Can you work these out from the model? Positions are in its coordinate system, mm. Give positions to 0.01 mm unless a question says otherwise; leave off trailing zeros. Order: outer loops, then holes, each group sorted by start corner. A loop starts at its lowest first (then second) coordinate and runs counter-clockwise, first axis right, second up. Notation, with made-up numbers: M 70,-33.75 L 108,-33.75 A29 cw 108,-1.75 Z; hole C 9.25,-19 d4. An arc over 180 degrees is marked long. Use one line per item in the form item = value. Start each with the question number.
1. I want a section at A-A, the plane z = 66.5. List the corners of the cut face in (x, y) for me.
2. I want a section at C-C, the plane x = 88.5. Count the separate pieces of the cut face and the enclosed holes in it, and give its area (3 significant figures).
3. Will these pins go through, and if not, where does the flat tip stop? P1, Ø2, axis at y = 2.5, z = 90.5, coming from the -X side; P2, Ø4, axis at x = -77.78, z = 77.78, coming from the +Y side; P3, Ø1, axis at y = 3.5, z = -82.5, coming from the -X side; P4, Ø1.5, axis at x = -49.5, y = 1, coming from the +Z side.
4. I want a section at B-B, the plane x = 8.5. List the corners of the cut face in (y, z) for me, and give its area (3 significant figures).
5. I need wall thicknesses on L1, parallel to Z at x = 86, y = 2; L2, parallel to Z at x = 0.5, y = 2; L3, parallel to X at y = 1.5, z = 76.5. Which ranges of each line are inside material? Lowest first, please.
```python
from build123d import *

# Parameters (mm, degrees)
SKETCH1_R           = 125
SKETCH1_R_2         = 1.5
BOSS_EXTRUDE1_DEPTH = 6


with BuildPart() as part:
    # Sketch1 → Boss-Extrude1 (new body)
    with BuildSketch(Plane(origin=(0, 0, 0), x_dir=(1, 0, 0), z_dir=(0, 1, 0))):
        with Locations(Location((0, 0, 0), (0, 0, 270))):
            Circle(SKETCH1_R)
        with Locations(Location((0, -110, 0), (0, 0, 270))):
            Circle(SKETCH1_R_2, mode=Mode.SUBTRACT)
        with Locations(Location((77.781745931, -77.781745931, 0), (0, 0, 270))):
            Circle(SKETCH1_R_2, mode=Mode.SUBTRACT)
        with Locations(Location((110, 0, 0), (0, 0, 270))):
            Circle(SKETCH1_R_2, mode=Mode.SUBTRACT)
        with Locations(Location((77.781745931, 77.781745931, 0), (0, 0, 270))):
            Circle(SKETCH1_R_2, mode=Mode.SUBTRACT)
        with Locations(Location((0, 110, 0), (0, 0, 90))):
            Circle(SKETCH1_R_2, mode=Mode.SUBTRACT)
        with Locations(Location((-77.781745931, 77.781745931, 0), (0, 0, 90))):
            Circle(SKETCH1_R_2, mode=Mode.SUBTRACT)
        with Locations(Location((-110, 0, 0), (0, 0, 90))):
            Circle(SKETCH1_R_2, mode=Mode.SUBTRACT)
        with Locations(Location((-77.781745931, -77.781745931, 0), (0, 0, 90))):
            Circle(SKETCH1_R_2, mode=Mode.SUBTRACT)
        with BuildLine():
            ThreePointArc((93.976500469, 13.907456977), (-95, 0), (93.976500469, -13.907456977))
            add(Edge.make_bspline(
                [(93.976500469, -13.907456977), (92.072801417, -3.957394346), (79.998651047, 0)],
                knots=[0, 0, 0, 1, 1, 1], degree=2))
            add(Edge.make_bspline(
                [(93.976500469, 13.907456977), (92.072801417, 3.957394346), (79.998651047, 0)],
                knots=[0, 0, 0, 1, 1, 1], degree=2))
        make_face(mode=Mode.SUBTRACT)
    extrude(amount=BOSS_EXTRUDE1_DEPTH)


solid = part.part
```
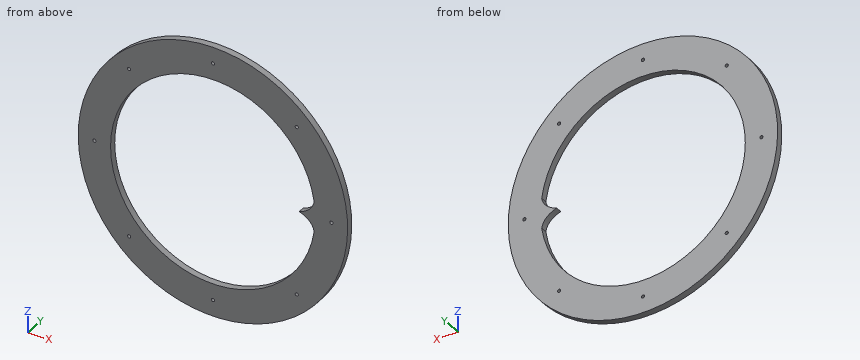
Check result:
q1.outline = M -105.84,0 L -67.84,0 L -67.84,6 L -105.84,6 Z; M 67.84,0 L 105.84,0 L 105.84,6 L 67.84,6 Z
q2.separate_pieces = 3
q2.enclosed_holes = 0
q2.area = 699 mm2
q3.P1 = -87.26
q3.P2 = 6
q3.P3 = -94.35
q3.P4 = 115.1
q4.outline = M 0,-124.71 L 6,-124.71 L 6,-94.62 L 0,-94.62 Z; M 0,94.62 L 6,94.62 L 6,124.71 L 0,124.71 Z
q4.area = 361 mm2
q5.L1 = -90.71 to -40.36, -2.71 to 2.71, 40.36 to 90.71
q5.L2 = -125 to -111.41, -108.59 to -95, 95 to 108.59, 111.41 to 125
q5.L3 = -98.86 to -78.56, -77 to -56.33, 56.33 to 77, 78.56 to 98.86
